Here's the drawing with two shaded views (mm, measured from the low corner). I have some questions. Coordinates: 2 decimals unless noted, no trailing zeros. Write each loop counter-clockwise with the first axis right and the second up, starting at its lowest first coordinate (ties: lowest second). Pieces come first, ordered by that corner, then holes. Notation, with made-up numbers: (61, 53.25) -> (119, 53.25) arc R17 ccw to (119, 74.25) -> close; hole circle Ø11 at (85.25, -31.75). An arc over 180 degrees is marked (long way). Answer in a Markdown table with one row per item. Add a question column.
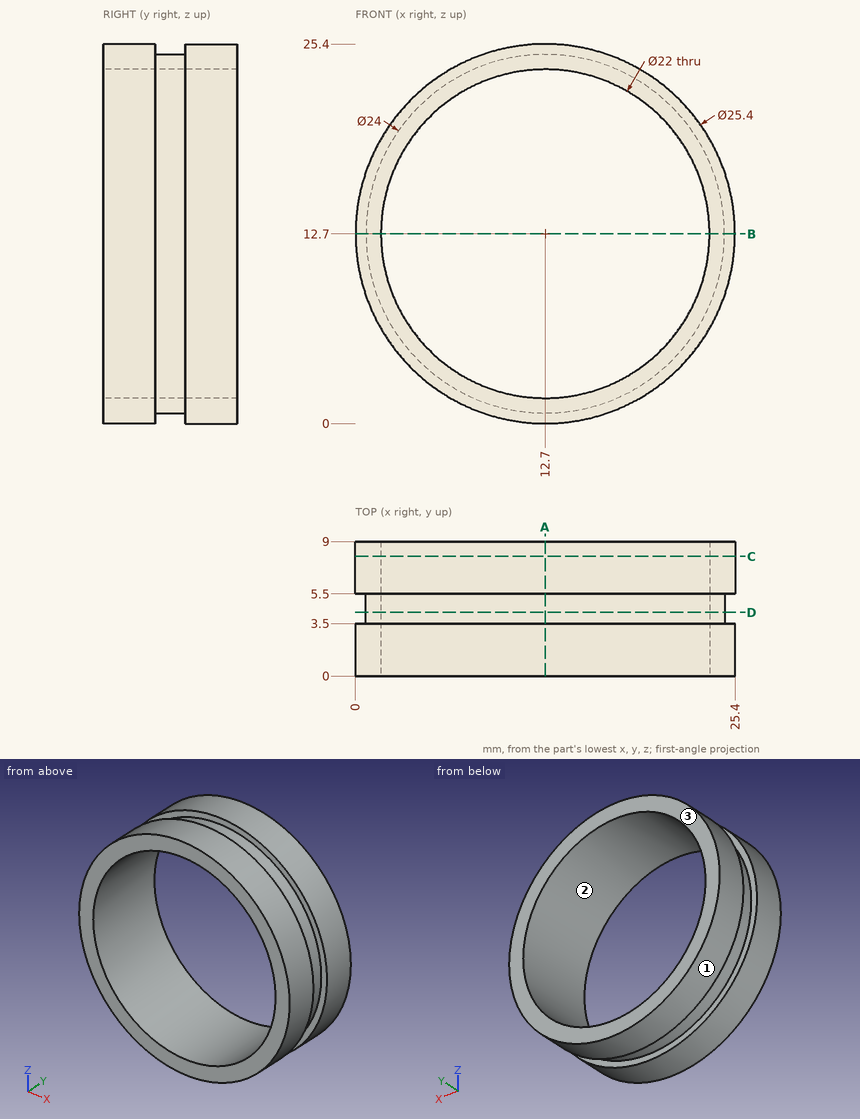
Q1. Imagine slicing it at D-D on y = 4.25. Please give me the cut outline in (x, z).
Q2. I need wall thicknesses on line 1 (Z direction, x = 12.7, y = 4); line 2 (Z direction, x = 14.5, y = 5); line 3 (X direction, y = 2.25, z = 8.75). Which ranges of each line are inside material? Lowest first, please. Write a range as [from, to].
Q3. Imagine slicing it at A-A on x = 12.7. Please give me the cut outline in (y, z), plus the area to 3 significant figures.
Q4. I'm going to push flat-ended pins straight in: P1, Ø5, axis at y = 7.5, z = 18.5, coming from the -X side; P2, Ø4, axis at x = 19.5, y = 3, coming from the -Z side; P3, Ø2, axis at y = 2, z = 22, coming from the -X side. Where does each tip first touch, or does it pass through?
Q5. Imagine slicing it at B-B on z = 12.7. Please give me the cut outline in (x, y), plus the area to 3 significant figures.
Q6. Imagine slicing it at C-C on y = 8. Please give me the cut outline in (x, z).
Q7. If we mould it in two halves opening along Z, with no side actions, what happens to the marked faces 1, 2 and 3? For each: pulls with the +Z half, pulls with the -Z half, needs draft (parallel to the pull), parting line crosses it, or undercut.
Result sheet:
| question | item | result |
|---|---|---|
| 1 | outline | circle Ø24 at (12.7, 12.7); hole circle Ø22 at (12.7, 12.7) |
| 2 | line 1 | z = [0.7, 1.7], [23.7, 24.7] |
| 2 | line 2 | z = [0.84, 1.85], [23.55, 24.56] |
| 2 | line 3 | x = [0.63, 2.43], [22.97, 24.77] |
| 3 | outline | (0, 0) -> (3.5, 0) -> (3.5, 0.7) -> (5.5, 0.7) -> (5.5, 0) -> (9, 0) -> (9, 1.7) -> (0, 1.7) -> close; (0, 23.7) -> (9, 23.7) -> (9, 25.4) -> (5.5, 25.4) -> (5.5, 24.7) -> (3.5, 24.7) -> (3.5, 25.4) -> (0, 25.4) -> close |
| 3 | area | 27.8 mm^2 |
| 4 | P1 | stops at x = 0.44 |
| 4 | P2 | stops at z = 0.94 |
| 4 | P3 | stops at x = 3.09 |
| 5 | outline | (0, 0) -> (1.7, 0) -> (1.7, 9) -> (0, 9) -> (0, 5.5) -> (0.7, 5.5) -> (0.7, 3.5) -> (0, 3.5) -> close; (23.7, 0) -> (25.4, 0) -> (25.4, 3.5) -> (24.7, 3.5) -> (24.7, 5.5) -> (25.4, 5.5) -> (25.4, 9) -> (23.7, 9) -> close |
| 5 | area | 27.8 mm^2 |
| 6 | outline | circle Ø25.4 at (12.7, 12.7); hole circle Ø22 at (12.7, 12.7) |
| 7 | face 1 | parting line crosses it |
| 7 | face 2 | undercut |
| 7 | face 3 | needs draft |
